Check sheet for the drawn part. Datum: minimum x, y, z corner. Units: mm. A direction names the side the tool comes from. Coordinates: 2 decimals unless noted, no trailing zeros. Write each loop counter-clockwise with the first axis right and the second up, starting at its lowest first coordinate (ties: lowest second). Pieces come first, ordered by that corner, then holes. Notation, with made-up numbers: M -19.5,22.25 L 15.5,22.25 A21 ccw 15.5,45.25 Z; hole C 64.5,-9 d3. An arc over 180 degrees is marked long. Write item = value, one per line. Start each with the question number.
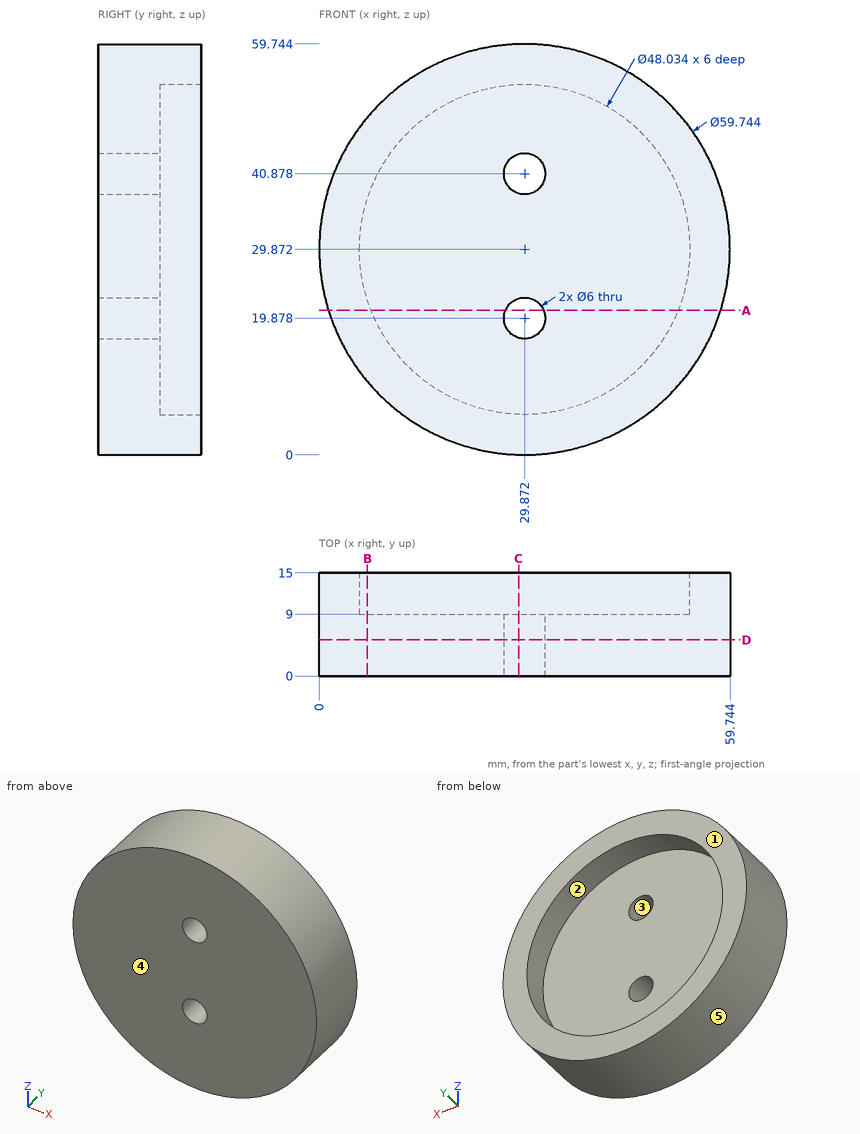
Q1. Cross-section at B-B on x = 7. Enter the section's corners in (y, z) (1 decimal).
Q2. Gauge pin test, flat ends, axial feed: pin 1 (8 mm diameter, centred on x = 40.5, y = 6, fed in from -Z) (1 decimal); pin 2 (8 mm diameter, centred on x = 42, y = 6, fed in from -Z); pin 3 (1 mm diameter, centred on y = 10.5, z = 46, fed in from +X). Record the tip position at first contact, or that the pin passes through.
Q3. Cross-section at A-A on z = 21. Enter the section's corners in (x, y).
Q4. Draft check along Z on the marked faces 3, 4 and 5. Enter one of: pulls with the +Z half, pulls with the -Z half, needs draft (parallel to the pull), parting line crosses it, or undercut.
Q5. Scan lines: L1, parallel to Z at x = 29.5, y = 7.25 (1 decimal); L2, parallel to Z at x = 31.5, y = 0.75 (1 decimal); L3, parallel to Z at x = 30, y = 14 (1 decimal). Record each from-to range of solid material in increasing order.
Q6. Cross-section at D-D on y = 5.25. Enter the section's corners in (x, z).
Q7. Set-up check for the marked faces 1 and 2: record each of +Z, -Z, +X, -X, +Y, -Y from which the full face is reachable in a straight line by a thin tool's end or side.
Q8. Cross-section at C-C on x = 29. Enter the section's corners in (y, z).
Values found:
q1.outline = M 0,10.7 L 15,10.7 L 15,22.5 L 9,22.5 L 9,37.2 L 15,37.2 L 15,49.1 L 0,49.1 Z
q2.pin_1 = 0.7
q2.pin_2 = 1.13
q2.pin_3 = 55.33
q3.outline = M 1.35,0 L 27.09,0 L 27.09,9 L 7.55,9 L 7.55,15 L 1.35,15 Z; M 32.65,0 L 58.4,0 L 58.4,15 L 52.19,15 L 52.19,9 L 32.65,9 Z
q4.face_3 = undercut
q4.face_4 = needs draft
q4.face_5 = parting line crosses it
q5.L1 = 0 to 16.9, 22.9 to 37.9, 43.9 to 59.7
q5.L2 = 0 to 17.4, 22.4 to 38.4, 43.4 to 59.7
q5.L3 = 0 to 5.9, 53.9 to 59.7
q6.outline = C 29.87,29.87 d59.74; hole C 29.87,19.88 d6; hole C 29.87,40.88 d6
q7.face_1 = +Z, -Z, +X, -X, +Y
q7.face_2 = +Y
q8.outline = M 0,0.01 L 15,0.01 L 15,5.87 L 9,5.87 L 9,17.01 L 0,17.01 Z; M 0,22.75 L 9,22.75 L 9,38.01 L 0,38.01 Z; M 0,43.75 L 9,43.75 L 9,53.87 L 15,53.87 L 15,59.73 L 0,59.73 Z
